Verification items for the finished model (mm, model axes). A direction names the side the tool comes from. Give positions to 0.01 mm unless a question says otherwise; leave off trailing zeros. Write each loop counter-clockwise with the first axis right and the second up, starting at its lowest first coordinate (ties: lowest second). Pieces come first, ordered by that corner, then holes. Notation, with made-up numbers: (1, 7) - (38, 7) arc R13 ccw to (38, 22) - close; hole circle Ø10 at (7.25, 66.25). An arc over 180 degrees is marked (long way). Put each result on its own line as item: value.
from build123d import *

# Parameters (mm, degrees)
SKETCH3_W           = 26.2
SKETCH3_H           = 16
SKETCH3_R           = 2.1
BOSS_EXTRUDE1_DEPTH = 1.5
BOSS_EXTRUDE2_START = -13.1
BOSS_EXTRUDE2_DEPTH = 25
CHAMFER1_SIZE       = 3
CHAMFER1_SIZE2      = 2.769187039
FILLET1_R           = 2


with BuildPart() as part:
    # Sketch3 → Boss-Extrude1 (new body)
    with BuildSketch(Plane.XY):
        with Locations((0, 47.9)):
            Rectangle(SKETCH3_W, SKETCH3_H)
        with Locations((8, 46)):
            Circle(SKETCH3_R, mode=Mode.SUBTRACT)
        with Locations((-8, 46)):
            Circle(SKETCH3_R, mode=Mode.SUBTRACT)
    extrude(amount=BOSS_EXTRUDE1_DEPTH)

    # Sketch4 → Boss-Extrude2 (add, symmetric)
    with BuildSketch(Plane(origin=(13.1, 0, 0), x_dir=(0, 0, -1), z_dir=(1, 0, 0)).offset(BOSS_EXTRUDE2_START)):
        Polygon((-1.5, 55.9), (-21.5, 54.150226729), (-21.5, 52.150226729), (-1.5, 53.9), align=None)
    extrude(amount=BOSS_EXTRUDE2_DEPTH, both=True)

    # Chamfer1
    chamfer1_edges = [part.edges().sort_by_distance(p)[0] for p in [
        (0, 53.9, 1.5),
    ]]
    chamfer1_side = [part.faces().sort_by_distance(p)[0] for p in [
        (0, 46.973543536, 1.5),
    ]]
    chamfer(chamfer1_edges, length=CHAMFER1_SIZE, length2=CHAMFER1_SIZE2, reference=chamfer1_side[0])

    # Fillet1
    fillet1_edges = [part.edges().sort_by_distance(p)[0] for p in [
        (-25, 54.9, 1.5),
        (-25, 53.150226729, 21.5),
        (25, 54.9, 1.5),
        (25, 53.150226729, 21.5),
        (13.1, 39.9, 0.75),
        (-13.1, 39.9, 0.75),
    ]]
    fillet(fillet1_edges, radius=FILLET1_R)


solid = part.part
Q1. Section check A-A, the plane y = 46. Record the cut outline in (x, z), plus the area to 3 significant figures.
Answers follow:
outline: (-13.1, 0) - (-10.1, 0) - (-10.1, 1.5) - (-13.1, 1.5) - close; (-5.9, 0) - (5.9, 0) - (5.9, 1.5) - (-5.9, 1.5) - close; (10.1, 0) - (13.1, 0) - (13.1, 1.5) - (10.1, 1.5) - close
area: 26.7 mm2
Q2. Set-up check for faces 1 (the face through (-13.1, 50, 1)), 2 (the face through (-18, 55, 1.5)), 3 (the face through (-12.53, 40.5, 0.76)), 4 (the face through (18, 55, 1.5)), 5 (the face through (13.1, 50, 1)): record each of +Z, -Z, +X, -X, +Y, -Y from which the full face is reachable in a straight line by a thin tool's end or side.
Answers follow:
face 1: -Z, -X, -Y
face 2: -Z, -X, +Y, -Y
face 3: +Z, -Z, -X, -Y
face 4: -Z, +X, +Y, -Y
face 5: -Z, +X, -Y
Q3. Section check B-B, the plane x = -8. Record the cut outline in (y, z).
Answers follow:
outline: (39.9, 0) - (43.9, 0) - (43.9, 1.5) - (39.9, 1.5) - close; (48.1, 0) - (55.9, 0) - (55.9, 1.5) - (54.15, 21.5) - (52.15, 21.5) - (53.66, 4.26) - (50.9, 1.5) - (48.1, 1.5) - close
Q4. Release check for a two-part mould opening along Z. For faces 6 (the face through (0.2, 52.3, 2.9)), 7 (the face through (-25, 54, 12)), 8 (the face through (0.35, 55.037, 11.36)) record: released by +Z, released by -Z, zero draft, split by the parting line, or undercut.
Answers follow:
face 6: undercut
face 7: zero draft
face 8: released by +Z
Q5. Section check C-C, the plane z = 11.75. Record the cut outline in (x, y), plus the area to 3 significant figures.
Answers follow:
outline: (-25, 53) - (25, 53) - (25, 55) - (-25, 55) - close
area: 100 mm2
Q6. Go/stop test with flat-tipped pins: pin 1 Ø2 at (x, y) = (16, 54.5) entering from -Z; pin 2 Ø2 at (y, z) = (46.5, 1.5) entering from +X; pin 3 Ø5 at (x, z) = (-15, 16) entering from -Y; pin 4 Ø2.5 at (x, y) = (8, 46) entering from +Z. Record where each tip stops, or that it passes through.
Answers follow:
pin 1: stops at z = 1.5
pin 2: stops at x = 13.1
pin 3: stops at y = 52.41
pin 4: passes through
Q7. Section check D-D, the plane y = 49.5. Record the cut outline in (x, z), plus the area to 3 significant figures.
Answers follow:
outline: (-13.1, 0) - (13.1, 0) - (13.1, 1.5) - (-13.1, 1.5) - close
area: 39.3 mm2
Q8. Scan lines: line 1 along Y through (x, z) = (-8, 0.7); line 2 along Z through (x, y) = (-12, 43.75); line 3 along X through (y, z) = (52.25, 2.5). Record each from-to range of solid material in increasing order.
Answers follow:
line 1: y = 39.9 to 43.9, 48.1 to 55.9
line 2: z = 0 to 1.5
line 3: x = -13.1 to 13.1
